```python
from build123d import *

# Parameters (mm, degrees)
SKETCH_1_W          = 130
SKETCH_1_H          = 130
EXTRUDE_1_DEPTH     = 3
SKETCH_2_R          = 2.6
CUT_EXTRUDE_1_DEPTH = 92.972822073
SKETCH_4_W          = 20.5
SKETCH_4_H          = 20.5
CUT_EXTRUDE_2_DEPTH = 1
SKETCH_5_W          = 89
SKETCH_5_H          = 5.1
SKETCH_5_W_2        = 5.1
SKETCH_5_H_2        = 89
CUT_EXTRUDE_3_DEPTH = 1
CHAMFER_1_SIZE      = 0.2
FILLET_1_R          = 0.5
FILLET_2_R          = 1


with BuildPart() as part:
    # 草图1 → 凸台-拉伸1 (new body)
    with BuildSketch(Plane(origin=(0, 0, 0), x_dir=(1, 0, 0), z_dir=(0, 1, 0))):
        Rectangle(SKETCH_1_W, SKETCH_1_H)
    extrude(amount=EXTRUDE_1_DEPTH)

    # 草图2 → 切除-拉伸1 (cut, through all)
    with BuildSketch(Plane(origin=(0, 3, 0), x_dir=(1, 0, 0), z_dir=(0, 1, 0))):
        with Locations(Location((52.5, 52.5, 0), (0, 0, 270))):
            Circle(SKETCH_2_R)
        with Locations(Location((52.5, -52.5, 0), (0, 0, 270))):
            Circle(SKETCH_2_R)
        with Locations(Location((-52.5, -52.5, 0), (0, 0, 270))):
            Circle(SKETCH_2_R)
        with Locations(Location((-52.5, 52.5, 0), (0, 0, 270))):
            Circle(SKETCH_2_R)
    extrude(amount=-CUT_EXTRUDE_1_DEPTH, mode=Mode.SUBTRACT)

    # 草图4 → 切除-拉伸2 (cut)
    with BuildSketch(Plane(origin=(0, 3, 0), x_dir=(1, 0, 0), z_dir=(0, 1, 0))):
        with Locations((54.75, 54.75)):
            Rectangle(SKETCH_4_W, SKETCH_4_H)
        with Locations((54.75, -54.75)):
            Rectangle(SKETCH_4_W, SKETCH_4_H)
        with Locations((-54.75, -54.75)):
            Rectangle(SKETCH_4_W, SKETCH_4_H)
        with Locations((-54.75, 54.75)):
            Rectangle(SKETCH_4_W, SKETCH_4_H)
    extrude(amount=-CUT_EXTRUDE_2_DEPTH, mode=Mode.SUBTRACT)

    # 草图5 → 切除-拉伸3 (cut)
    with BuildSketch(Plane(origin=(0, 3, 0), x_dir=(1, 0, 0), z_dir=(0, 1, 0))):
        with Locations((0, 62.45)):
            Rectangle(SKETCH_5_W, SKETCH_5_H)
        with Locations((62.45, 0)):
            Rectangle(SKETCH_5_W_2, SKETCH_5_H_2)
        with Locations((0, -62.45)):
            Rectangle(SKETCH_5_W, SKETCH_5_H)
        with Locations((-62.45, 0)):
            Rectangle(SKETCH_5_W_2, SKETCH_5_H_2)
    extrude(amount=-CUT_EXTRUDE_3_DEPTH, mode=Mode.SUBTRACT)

    # 倒角1
    chamfer_1_edges = [part.edges().sort_by_distance(p)[0] for p in [
        (65, 1, 65),
        (-65, 1, 65),
        (-65, 1, -65),
        (65, 1, -65),
    ]]
    chamfer(chamfer_1_edges, length=CHAMFER_1_SIZE)

    # 圆角1
    # the kernel refuses this fillet: 0.5 mm, written as the material it takes off along each edge
    with BuildSketch(Plane(origin=(-65, 0, 66.05), x_dir=(1, 0, 0), z_dir=(0, 0, -1)), Plane(origin=(66.05, 0, 65), x_dir=(0, 0, -1), z_dir=(-1, 0, 0)), Plane(origin=(65, 0, -66.05), x_dir=(-1, 0, 0), z_dir=(0, 0, 1))) as fillet_1_piece_1:
        with BuildLine():
            CenterArc((FILLET_1_R, -FILLET_1_R), FILLET_1_R, 90, 90)
            Line((0, -FILLET_1_R), (0, 0))
            Line((0, 0), (FILLET_1_R, 0))
        make_face()
    extrude(amount=132.1, mode=Mode.SUBTRACT)
    with BuildSketch(Plane(origin=(-66.05, 0, -65), x_dir=(0, 1, 0), z_dir=(1, 0, 0))) as fillet_1_piece_2:
        with BuildLine():
            CenterArc((FILLET_1_R, FILLET_1_R), FILLET_1_R, 180, 90)
            Line((0, FILLET_1_R), (0, 0))
            Line((0, 0), (FILLET_1_R, 0))
        make_face()
    extrude(amount=132.1, mode=Mode.SUBTRACT)

    # 圆角2
    fillet_2_edges = [part.edges().sort_by_distance(p)[0] for p in [
        (-44.5, 2.5, -59.9),
        (44.5, 2.5, -59.9),
        (59.9, 2.5, -44.5),
        (59.9, 2.5, 44.5),
        (44.5, 2.5, 59.9),
        (-44.5, 2.5, 59.9),
        (-59.9, 2.5, 44.5),
        (-59.9, 2.5, -44.5),
        (-44.5, 2.5, -44.5),
        (-44.5, 2.5, 44.5),
        (44.5, 2.5, 44.5),
        (44.5, 2.5, -44.5),
    ]]
    fillet(fillet_2_edges, radius=FILLET_2_R)


solid = part.part
```
Part model, mm, in its own coordinate system. A direction names the side the tool comes from. Round coordinates to 2 decimals unless told otherwise and drop trailing zeros. Write each loop counter-clockwise with the first axis right and the second up, starting at its lowest first coordinate (ties: lowest second). Pieces come first, ordered by that corner, then holes.
Item 1: Which spindle directions (+Z, -Z, +X, -X, +Y, -Y) get a long thin tool onto all of the face, cutting with end or side? Do faces 3 (the cylindrical face through (-52.4, 1, 49.9)), 4 (the flat face through (0, 2, -63)). Say none if no direction does.
Results:
face 3: +Y, -Y
face 4: +Y
Item 2: Cut at D-D, the plane x = -29.5. Give the cut face in (y, z), plus the area to 3 significant figures.
Results:
outline: (0, -64.5) arc R0.5 ccw to (0.5, -65) - (2, -65) - (2, -59.9) - (3, -59.9) - (3, 59.9) - (2, 59.9) - (2, 65) - (0.5, 65) arc R0.5 ccw to (0, 64.5) - close
area: 380 mm2
Item 3: Cut at A-A, the plane x = 52.5. Give the cut face in (y, z), plus the area to 3 significant figures.
Results:
outline: (0, -64.5) arc R0.5 ccw to (0.5, -65) - (2, -65) - (2, -55.1) - (0, -55.1) - close; (0, -49.9) - (2, -49.9) - (2, -44.5) - (3, -44.5) - (3, 44.5) - (2, 44.5) - (2, 49.9) - (0, 49.9) - close; (0, 55.1) - (2, 55.1) - (2, 65) - (0.5, 65) arc R0.5 ccw to (0, 64.5) - close
area: 328 mm2
Item 4: Probe L1, parallel to X at y = 0.7, z = -52.5; L2, parallel to Y at x = -46.5, z = -52; L3, parallel to Z at x = 11, y = 2.4. List the from-to ranges inside material, lowest first.
Results:
L1: x = -65 to -55.1, -49.9 to 49.9, 55.1 to 65
L2: y = 0 to 2
L3: z = -59.9 to 59.9
Item 5: Drop flat-ended pins along their axis: pin 1 Ø0.8 at (x, y) = (14, 2.5) entering from +Z; pin 2 Ø1.1 at (x, y) = (9.5, 2.5) entering from -Z; pin 3 Ø0.5 at (x, y) = (54, 2.5) entering from -Z; pin 4 Ø0.8 at (x, y) = (49, 2.5) entering from +Z. Give the stop position or say it passes through.
Results:
pin 1: stops at z = 59.9
pin 2: stops at z = -65
pin 3: stops at z = -44.5
pin 4: stops at z = 44.5
Item 6: Cut at C-C, the plane z = -57. Give the cut face in (x, y), plus the area to 3 significant figures.
Results:
outline: (-65, 0.5) arc R0.5 ccw to (-64.5, 0) - (64.5, 0) arc R0.5 ccw to (65, 0.5) - (65, 2) - (44.5, 2) - (44.5, 3) - (-44.5, 3) - (-44.5, 2) - (-65, 2) - close
area: 349 mm2
Item 7: Two-plate mould, pull along Z, no slides. Class faces 1 (the cylindrical face through (52.6, 1, -55.1)), 2 (the flat face through (-1, 0, -1)): +Z half, -Z half, draft (parallel to the pull), parting line (faces both ways), or undercut.
Results:
face 1: undercut
face 2: draft
Item 8: Cut at B-B, the plane z = 52.5. Give the cut face in (x, y).
Results:
outline: (-65, 0.5) arc R0.5 ccw to (-64.5, 0) - (-55.1, 0) - (-55.1, 2) - (-65, 2) - close; (-49.9, 0) - (49.9, 0) - (49.9, 2) - (44.5, 2) - (44.5, 3) - (-44.5, 3) - (-44.5, 2) - (-49.9, 2) - close; (55.1, 0) - (64.5, 0) arc R0.5 ccw to (65, 0.5) - (65, 2) - (55.1, 2) - close
